Geometry: final body of the model. Coordinates: model frame, mm. Face numbers are marked on the shaded views. Give positions to 0.01 mm unless a question says otherwise; leave off trailing zeros. Write each loop counter-clockwise with the first axis right and the second up, starting at its lowest first coordinate (ties: lowest second). Pieces come first, ordered by that corner, then holes. Notation, with made-up numbers: (71.25, -17.75) - (98.25, -17.75) arc R29 ccw to (98.25, 8.25) - close; hole circle Ø5 at (-11, -38.75). An arc over 180 degrees is marked (long way). Use CSV: the item, a comma, the result in double quotes. Start each with the question number.
(1) Section B-B on y = 9.25. Output: boundary loops of the cut face in (x, z) (3 decimals).
(2) First-contact query: pin 1 Ø5.5 at (y, z) = (3, 44.5) entering from -X; pin 2 Ø6 at (y, z) = (7.5, 266.5) entering from +X; pin 3 Ø14.5 at (x, z) = (5.75, 117.28) entering from +Y; pin 4 Ø6 at (y, z) = (4.5, 221) entering from -X. Flat tips, straight axial feed; report the tip coordinate or a pass-through.
(3) Section D-D on x = 127.5. Output: boundary loops of the cut face in (y, z), and give its area (3 significant figures).
(4) Section C-C on z = 44. Output: boundary loops of the cut face in (x, y), and give its area (3 significant figures).
(5) Draft query along Y for the marked faces 1 and 2. Return one class per face: released by +Y, released by -Y, zero draft, split by the parting line, or undercut.
(6) Section A-A on x = 4.5. Output: boundary loops of the cut face in (y, z), and give its area (3 significant figures).
(7) Line query: probe 1 along Z at (x, y) = (10.5, 1); probe 2 along Z at (x, y) = (-5, 1.5); probe 3 along X at (y, z) = (7, 157.5). Output: solid intervals per line, ascending. Write a range as [from, to].
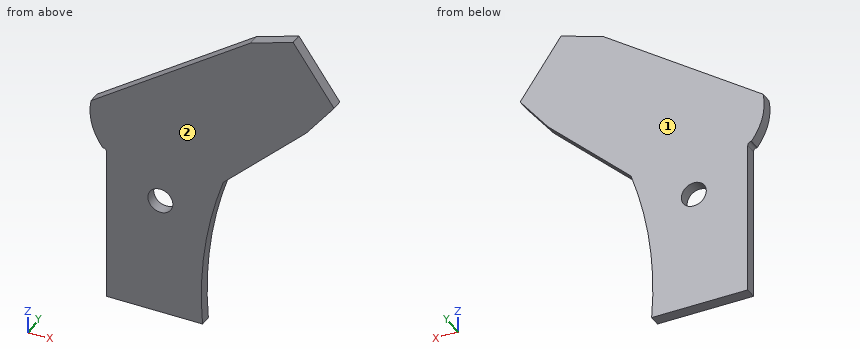
from build123d import *

# Parameters (mm, degrees)
SKETCH1_R           = 7.9375
BOSS_EXTRUDE1_DEPTH = 11.1125
SKETCH2_R           = 12.20390625
CUT_EXTRUDE1_DEPTH  = 11.1125


with BuildPart() as part:
    # Sketch1 → Boss-Extrude1 (new body)
    with BuildSketch(Plane(origin=(0, 0, 0), x_dir=(1, 0, 0), z_dir=(0, 1, 0))):
        with BuildLine():
            Line((47.0296875, 0), (-47.0296875, 0))
            Line((-47.0296875, 0), (-47.0296875, -152.5984375))
            ThreePointArc((-47.0296875, -152.5984375), (-47.95962347, -154.84350153), (-50.2046875, -155.7734375))
            Line((-50.2046875, -155.7734375), (-50.6015625, -155.7734375))
            ThreePointArc((-50.6015625, -155.7734375), (-61.399867308, -177.531283173), (-62.1109375, -201.8109375))
            Line((-62.1109375, -201.8109375), (93.937526937, -311.077248625))
            Line((93.937526937, -311.077248625), (135.682650242, -324.803661369))
            Line((135.682650242, -324.803661369), (175.746964321, -267.585891076))
            Line((175.746964321, -267.585891076), (148.570682499, -233.053016406))
            Line((148.570682499, -233.053016406), (67.2703125, -155.7734375))
            ThreePointArc((67.2703125, -155.7734375), (49.00058662, -78.945623418), (47.0296875, 0))
        make_face()
        with Locations((5.7546875, -117.2765625)):
            Circle(SKETCH1_R, mode=Mode.SUBTRACT)
    extrude(amount=BOSS_EXTRUDE1_DEPTH)

    # Sketch2 → Cut-Extrude1 (cut)
    with BuildSketch(Plane(origin=(0, 11.1125, 0), x_dir=(1, 0, 0), z_dir=(0, 1, 0))):
        with Locations((5.7546875, -117.2765625)):
            Circle(SKETCH2_R)
    extrude(amount=-CUT_EXTRUDE1_DEPTH, mode=Mode.SUBTRACT)


solid = part.part
Check values:
1,outline,"(-62.111, 201.811) arc R56.744 ccw to (-50.602, 155.773) - (-50.205, 155.773) arc R3.175 cw to (-47.03, 152.598) - (-47.03, 0) - (47.03, 0) arc R379.433 cw to (67.27, 155.773) - (148.571, 233.053) - (175.747, 267.586) - (135.683, 324.804) - (93.938, 311.077) - close; hole circle Ø24.408 at (5.755, 117.277)"
2,pin 1,"stops at x = -47.03"
2,pin 2,"stops at x = 175.75"
2,pin 3,"passes through"
2,pin 4,"stops at x = -38.99"
3,outline,"(0, 213.02) - (11.11, 213.02) - (11.11, 322.11) - (0, 322.11) - close"
3,area,"1,210 mm²"
4,outline,"(-47.03, 0) - (46.09, 0) - (46.09, 11.11) - (-47.03, 11.11) - close"
4,area,"1,030 mm²"
5,face 1,"released by +Y"
5,face 2,"released by -Y"
6,outline,"(0, 0) - (11.11, 0) - (11.11, 105.14) - (0, 105.14) - close; (0, 129.42) - (11.11, 129.42) - (11.11, 248.45) - (0, 248.45) - close"
6,area,"2,490 mm²"
7,probe 1,"z = [0, 106.03], [128.52, 252.65]"
7,probe 2,"z = [0, 111.51], [123.04, 241.8]"
7,probe 3,"x = [-51.93, 69.09]"
